Verification items for this drawing (mm, ordinates from the low corner). A direction names the side the tool comes from. Give positions to 0.01 mm unless a question says otherwise; leave off trailing zeros. Write each loop counter-clockwise with the first axis right and the second up, starting at its lowest first coordinate (ties: lowest second). Pieces come first, ordered by that corner, then holes. Notation, with made-up numbers: (17.25, 5.5) -> (67.25, 5.5) arc R15 ccw to (67.25, 14.5) -> close; hole circle Ø9 at (-31, 9). An arc over 180 degrees is marked (long way). Write item = value, one per line.
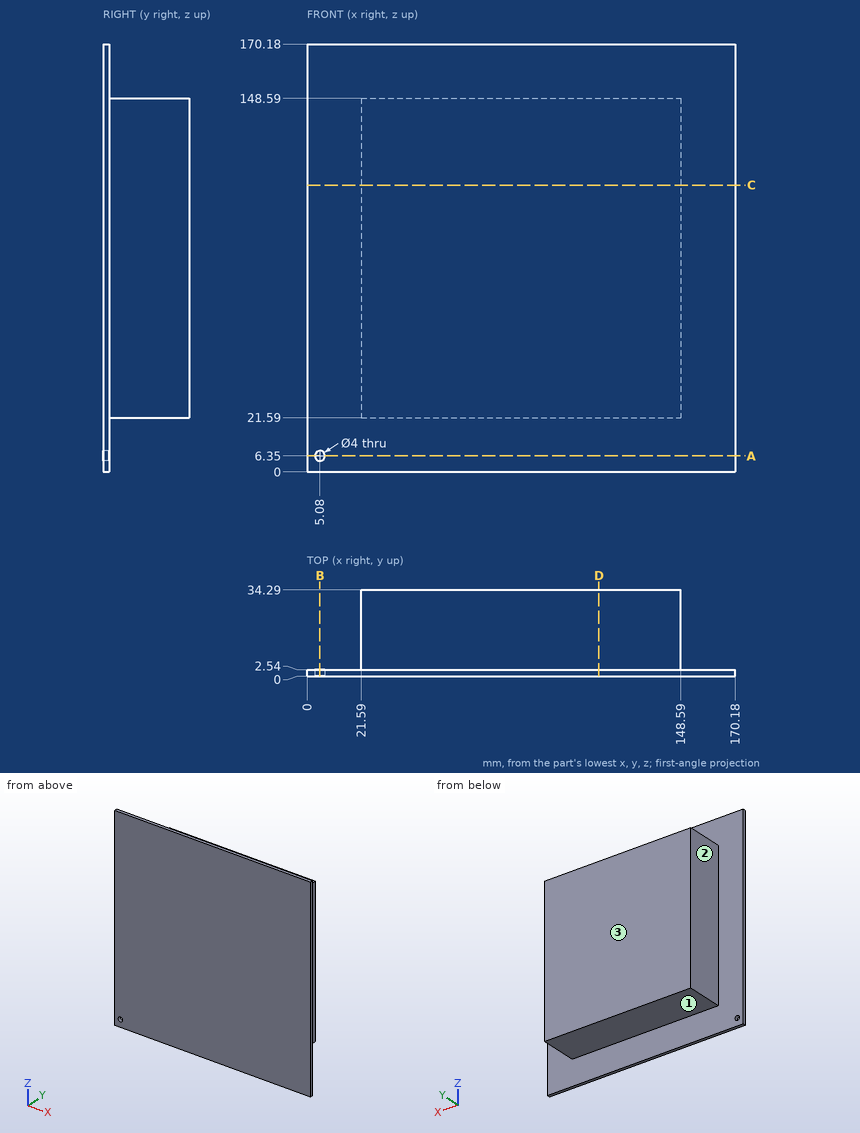
Item 1: Material ranges on line 1 (Z direction, x = 5.08, y = 0.95); line 2 (Z direction, x = 46, y = 33), recorded low to high.
Response values:
line_1 = 0 to 4.35, 8.35 to 170.18
line_2 = 21.59 to 148.59
Item 2: Sectioned sample at D-D on x = 116. Record the cut outline in (y, z), then the cut area to 3 significant figures.
Response values:
outline = (0, 0) -> (2.54, 0) -> (2.54, 21.59) -> (34.29, 21.59) -> (34.29, 148.59) -> (2.54, 148.59) -> (2.54, 170.18) -> (0, 170.18) -> close
area = 4,460 mm^2
Item 3: Sectioned sample at A-A on z = 6.35. Record the cut outline in (x, y).
Response values:
outline = (0, 0) -> (3.08, 0) -> (3.08, 2.54) -> (0, 2.54) -> close; (7.08, 0) -> (170.18, 0) -> (170.18, 2.54) -> (7.08, 2.54) -> close
Item 4: Sectioned sample at C-C on z = 114. Record the cut outline in (x, y).
Response values:
outline = (0, 0) -> (170.18, 0) -> (170.18, 2.54) -> (148.59, 2.54) -> (148.59, 34.29) -> (21.59, 34.29) -> (21.59, 2.54) -> (0, 2.54) -> close
Item 5: Go/stop test with flat-tipped pins: P1, Ø12, axis at x = 110.5, y = 17, coming from the -Z side; P2, Ø10, axis at y = 12.5, z = 81, coming from the +X side; P3, Ø8, axis at x = 58.5, y = 27.5, coming from the +Z side. Record where each tip stops, or that it passes through.
Response values:
P1 = 21.59
P2 = 148.59
P3 = 148.59
Item 6: Set-up check for the marked faces 1, 2 and 3: record each of +Z, -Z, +X, -X, +Y, -Y from which the full face is reachable in a straight line by a thin tool's end or side.
Response values:
face_1 = -Z, +X, -X, +Y
face_2 = +Z, -Z, -X, +Y
face_3 = +Z, -Z, +X, -X, +Y
Item 7: Sectioned sample at B-B on x = 5.08. Record the cut outline in (y, z), then the cut area to 3 significant figures.
Response values:
outline = (0, 0) -> (2.54, 0) -> (2.54, 4.35) -> (0, 4.35) -> close; (0, 8.35) -> (2.54, 8.35) -> (2.54, 170.18) -> (0, 170.18) -> close
area = 422 mm^2
